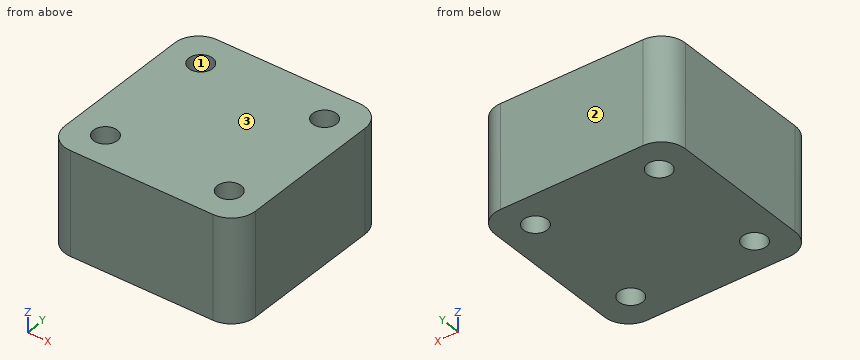
```python
from build123d import *

# Parameters (mm, degrees)
ESBO_O1_W                = 48
ESBO_O1_H                = 48
RESSALTO_EXTRUS_O1_DEPTH = 26
ESBO_O3_R                = 3
CORTE_EXTRUS_O2_DEPTH    = 27
FILETE2_R                = 6


with BuildPart() as part:
    # Esboço1 → Ressalto-extrusão1 (new body)
    with BuildSketch(Plane.XY):
        Rectangle(ESBO_O1_W, ESBO_O1_H)
    extrude(amount=RESSALTO_EXTRUS_O1_DEPTH)

    # Esboço3 → Corte-extrusão2 (cut, through all)
    with BuildSketch(Plane.XY.offset(26)):
        with Locations((-15.6, -15.6)):
            Circle(ESBO_O3_R)
        with Locations((-15.6, 15.6)):
            Circle(ESBO_O3_R)
        with Locations((15.6, -15.6)):
            Circle(ESBO_O3_R)
        with Locations((15.6, 15.6)):
            Circle(ESBO_O3_R)
    extrude(amount=-CORTE_EXTRUS_O2_DEPTH, mode=Mode.SUBTRACT)

    # Filete2
    filete2_edges = [part.edges().sort_by_distance(p)[0] for p in [
        (24, -24, 13),
        (-24, -24, 13),
        (-24, 24, 13),
        (24, 24, 13),
    ]]
    fillet(filete2_edges, radius=FILETE2_R)


solid = part.part
```
Part model, mm, in its own coordinate system. Face numbers are marked on the shaded views. Coordinates: 2 decimals unless noted, no trailing zeros. Order: outer loops, then holes, each group sorted by start corner. A loop starts at its lowest first (then second) coordinate and runs counter-clockwise, first axis right, second up. Notation, with made-up numbers: (-7.5, 26) - (50.5, 26) arc R26 cw to (50.5, 54) - close; hole circle Ø5 at (1.25, 36). An arc over 180 degrees is marked (long way). Return JSON: item names as keys, results as strings. Group by question number.
Item 1: Drill centre lines: probe 1 along X at (y, z) = (-15.5, 17.5); probe 2 along X at (y, z) = (-17, 6.5). Where is each one in solid material? Low to high. Write a range as from..to.
Item 2: Pull direction Y, two halves, no side cores. Call the marked faces 1, 2 and 3: pulls with the +Y half, pulls with the -Y half, needs draft (parallel to the pull), parting line crosses it, or undercut.
Item 3: Cut at A-A (x = 15.6). List the corners of the cut face in (y, z).
Item 4: Pin check, flat tip, straight feed: pin 1 (5 mm diameter, centred on x = 15.6, y = -15.6, fed in from +Z). Stop position of the tip, or through.
Item 5: Cut at B-B (z = 15.75). List the corners of the cut face in (x, y).
Check values:
{
 "1": {"probe 1": "x = -24..-18.6, -12.6..12.6, 18.6..24", "probe 2": "x = -24..-18.25, -12.95..12.95, 18.25..24"},
 "2": {"face 1": "undercut", "face 2": "pulls with the +Y half", "face 3": "needs draft"},
 "3": {"outline": "(-24, 0) - (-18.6, 0) - (-18.6, 26) - (-24, 26) - close; (-12.6, 0) - (12.6, 0) - (12.6, 26) - (-12.6, 26) - close; (18.6, 0) - (24, 0) - (24, 26) - (18.6, 26) - close"},
 "4": {"pin 1": "passes through"},
 "5": {"outline": "(-24, -18) arc R6 ccw to (-18, -24) - (18, -24) arc R6 ccw to (24, -18) - (24, 18) arc R6 ccw to (18, 24) - (-18, 24) arc R6 ccw to (-24, 18) - close; hole circle Ø6 at (-15.6, -15.6); hole circle Ø6 at (-15.6, 15.6); hole circle Ø6 at (15.6, -15.6); hole circle Ø6 at (15.6, 15.6)"}
}
